from build123d import *

# Parameters (mm, degrees)
F0_W      = 38.8747
F0_H      = 28.7528
F1_DEPTH  = 5.5245
F2_W      = 37.6047
F2_H      = 26.4668
F3_DEPTH  = 3.429
F4_W      = 1.27
F4_H      = 2.159
F5_DEPTH  = 1.27
F6_W      = 1.27
F6_H      = 2.159
F7_DEPTH  = 1.27
F8_W      = 1.27
F8_H      = 2.159
F9_DEPTH  = 1.27
F10_W     = 1.27
F10_H     = 2.159
F11_DEPTH = 1.27
F12_R     = 2.54
F13_DEPTH = 2.159
F14_R     = 1.4224
F15_DEPTH = 4.2555
F16_R     = 2.54
F17_DEPTH = 2.159
F18_R     = 1.4224
F19_DEPTH = 4.2555
F20_W     = 11.6967
F20_H     = 3.429
F21_DEPTH = 2.032


with BuildPart() as f1:
    # F0 (on Top) → F1 (new body)
    with BuildSketch(Plane.XY):
        Rectangle(F0_W, F0_H)
    extrude(amount=F1_DEPTH)

    # F2 (on face) → F3 (cut)
    with BuildSketch(Plane.XY.offset(5.5245)):
        Rectangle(F2_W, F2_H)
    extrude(amount=-F3_DEPTH, mode=Mode.SUBTRACT)

    # F4 (on face) → F5 (join)
    with BuildSketch(Plane.XZ.offset(-13.2334)):
        with Locations((-18.16735, 3.175)):
            Rectangle(F4_W, F4_H)
    extrude(amount=F5_DEPTH)

    # F6 (on face) → F7 (join)
    with BuildSketch(Plane(origin=(18.80235, 0, 0), x_dir=(0, -1, 0), z_dir=(-1, 0, 0))):
        with Locations((-12.5984, 3.175)):
            Rectangle(F6_W, F6_H)
    extrude(amount=F7_DEPTH)

    # F8 (on face) → F9 (join)
    with BuildSketch(Plane(origin=(0, -13.2334, 0), x_dir=(-1, 0, 0), z_dir=(0, 1, 0))):
        with Locations((-18.16735, 3.175)):
            Rectangle(F8_W, F8_H)
    extrude(amount=F9_DEPTH)

    # F10 (on face) → F11 (join)
    with BuildSketch(Plane(origin=(0, -13.2334, 0), x_dir=(-1, 0, 0), z_dir=(0, 1, 0))):
        with Locations((18.16735, 3.175)):
            Rectangle(F10_W, F10_H)
    extrude(amount=F11_DEPTH)

    # F12 (on face) → F13 (join)
    with BuildSketch(Plane.XY.offset(2.0955)):
        with Locations((-14.10335, 0)):
            Circle(F12_R)
    extrude(amount=F13_DEPTH)

    # F14 (on face) → F15 (cut, through all)
    with BuildSketch(Plane.XY.offset(4.2545)):
        with Locations((-14.10335, 0)):
            Circle(F14_R)
    extrude(amount=-F15_DEPTH, mode=Mode.SUBTRACT)

    # F16 (on face) → F17 (join)
    with BuildSketch(Plane.XY.offset(2.0955)):
        with Locations((14.10335, 0)):
            Circle(F16_R)
    extrude(amount=F17_DEPTH)

    # F18 (on face) → F19 (cut, through all)
    with BuildSketch(Plane.XY.offset(4.2545)):
        with Locations((14.10335, 0)):
            Circle(F18_R)
    extrude(amount=-F19_DEPTH, mode=Mode.SUBTRACT)

    # F20 (on face) → F21 (cut)
    with BuildSketch(Plane.XZ.offset(14.3764)):
        with Locations((0, 3.81)):
            Rectangle(F20_W, F20_H)
    extrude(amount=-F21_DEPTH, mode=Mode.SUBTRACT)


solid = f1.part
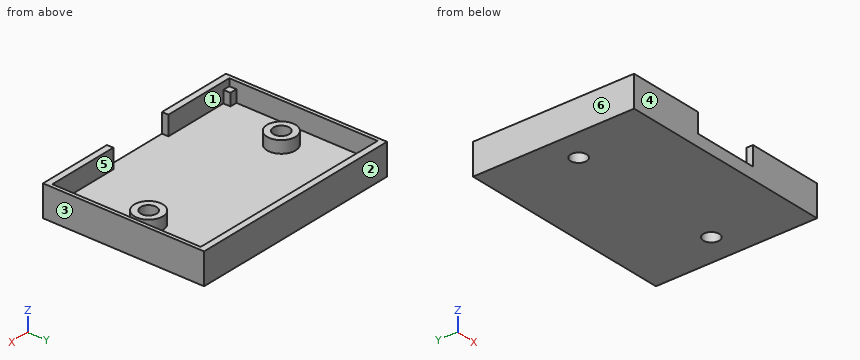
For this review, take the finished solid that the model builds, in its own axes (mm). Face numbers are marked on the shaded views. A direction names the side the tool comes from. Round coordinates to 2 decimals unless told otherwise and drop trailing zeros. Loops run counter-clockwise (first coordinate to the right, second up) from the corner with the lowest first, then second, coordinate; pieces in that order, holes last. Notation, with made-up numbers: (-23, 31.5) - (1, 31.5) arc R16 ccw to (1, 48.5) - close; hole circle Ø10 at (-11, -2). An arc over 180 degrees is marked (long way). One line per question, with ' | ' between items.
Q1. The part is to be moulded in two halves that separate along X. For the marked faces 3, 4, 5 and 6, say which applies: released by +X, released by -X, zero draft, split by the parting line, or undercut.
Taken from the geometry:
face 3: released by +X | face 4: zero draft | face 5: undercut | face 6: released by -X
Q2. Take a section at B-B (x = 6.5). Give the boundary of the cut face in (y, z), and give its area (3 significant figures).
Taken from the geometry:
outline: (-14.38, 0) - (14.38, 0) - (14.38, 5.52) - (13.23, 5.52) - (13.23, 2.1) - (-13.23, 2.1) - (-13.23, 5.52) - (-14.38, 5.52) - close | area: 68.1 mm²
Q3. For line 1 along Y through (x, z) = (-12, 3.2); line 2 along X through (y, z) = (-0.75, 4.7); line 3 along Y through (x, z) = (12, 4.35), list the stretches that pass through material, from the lowest coordinate up. Write a range as [from, to].
Taken from the geometry:
line 1: y = [-14.38, -13.23], [-1.42, 1.42], [13.23, 14.38] | line 2: x = [-19.44, -18.8], [18.8, 19.44] | line 3: y = [-14.38, -13.23], [13.23, 14.38]
Q4. Take a section at A-A (y = 0). Give the boundary of the cut face in (x, z).
Taken from the geometry:
outline: (-19.44, 0) - (-15.53, 0) - (-15.53, 4.25) - (-16.64, 4.25) - (-16.64, 2.1) - (-18.8, 2.1) - (-18.8, 5.52) - (-19.44, 5.52) - close; (-12.68, 0) - (12.68, 0) - (12.68, 4.25) - (11.56, 4.25) - (11.56, 2.1) - (-11.56, 2.1) - (-11.56, 4.25) - (-12.68, 4.25) - close; (15.53, 0) - (19.44, 0) - (19.44, 5.52) - (18.8, 5.52) - (18.8, 2.1) - (16.64, 2.1) - (16.64, 4.25) - (15.53, 4.25) - close
Q5. For pin 1 (8.5 mm diameter, centred on x = 1, y = -2.5, fed in from +Z); pin 2 (3.5 mm diameter, centred on x = 14.1, y = 0, fed in from +Z), all flat-tipped, find the tip position at first contact; note any pin that passes through.
Taken from the geometry:
pin 1: stops at z = 2.1 | pin 2: stops at z = 4.25
Q6. Take a section at C-C (y = 9.5). Give the boundary of the cut face in (x, z), and give its area (3 significant figures).
Taken from the geometry:
outline: (-19.44, 0) - (19.44, 0) - (19.44, 5.52) - (18.8, 5.52) - (18.8, 2.1) - (-18.8, 2.1) - (-18.8, 5.52) - (-19.44, 5.52) - close | area: 85.8 mm²
Q7. Tool access review of the marked faces 1 and 2: name each direction out of +Z, -Z, +X, -X, +Y, -Y from which nothing blocks a thin tool from reaching the whole face with its end or side.
Taken from the geometry:
face 1: +Z | face 2: +Z, -Z, +X, -X, +Y
Q8. Take a section at D-D (x = -16). Give the boundary of the cut face in (y, z).
Taken from the geometry:
outline: (-14.38, 0) - (14.38, 0) - (14.38, 5.52) - (13.23, 5.52) - (13.23, 2.1) - (1.69, 2.1) - (1.69, 4.25) - (-1.69, 4.25) - (-1.69, 2.1) - (-13.23, 2.1) - (-13.23, 5.52) - (-14.38, 5.52) - close
